Part print with two shaded views. Sizes in mm from the minimum x, y, z corner. A direction names the side the tool comes from. Coordinates: 2 decimals unless noted, no trailing zeros. Write each loop counter-clockwise with the first axis right and the second up, starting at its lowest first coordinate (ties: lowest second). Pieces come first, ordered by that corner, then holes. Notation, with made-up numbers: (11.5, 57.5) -> (67.5, 57.5) arc R23 ccw to (67.5, 69.5) -> close; hole circle Ø10 at (53.25, 25.25). An arc over 180 degrees is marked (long way). Write item = value, one per line. Start each with the question number.
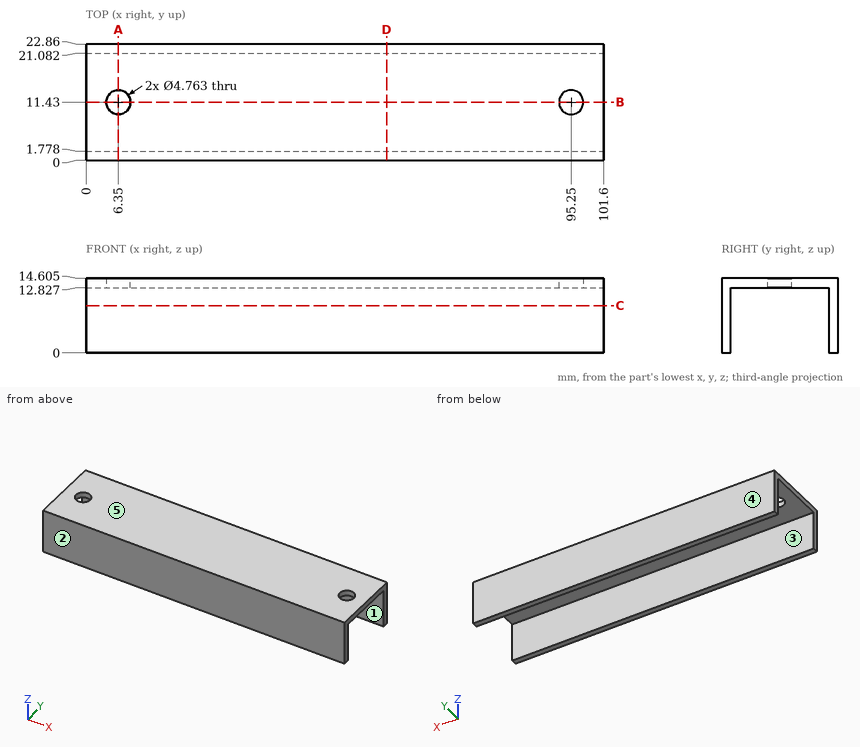
(1) 3-axis set-ups, long thin cutter, end or side, ignore diameter. For the marked faces 1 and 2: which of +Z, -Z, +X, -X, +Y, -Y reach the whole face in a straight line?
(2) Saw through at A-A (x = 6.35). Give the cut face in (y, z) (1 decimal).
(3) Saw through at B-B (y = 11.43). Give the cut face in (x, z) (1 decimal).
(4) Drop a flat-ended pin along its axis: pin 1 Ø5 at (x, y) = (65.5, 9.5) entering from -Z. Give the stop position or say it passes through.
(5) Saw through at D-D (x = 59). Give the cut face in (y, z) (1 decimal).
(6) Saw through at C-C (z = 9.25). Give the cut face in (x, y).
(7) Mould opens along Y. For the marked faces 3, 4 and 5 say: released by +Y, released by -Y, zero draft, split by the parting line, or undercut.
(8) Drill centre lines: line 1 along Y through (x, z) = (6.35, 14.2); line 2 along Y through (x, z) = (32.5, 7); line 3 along Z through (x, y) = (10, 9.75) (1 decimal). Where is each one in solid material? Low to high.
Returned:
q1.face_1 = -Z, +X, -X
q1.face_2 = +Z, -Z, +X, -X, -Y
q2.outline = (0, 0) -> (1.8, 0) -> (1.8, 12.8) -> (9, 12.8) -> (9, 14.6) -> (0, 14.6) -> close; (13.8, 12.8) -> (21.1, 12.8) -> (21.1, 0) -> (22.9, 0) -> (22.9, 14.6) -> (13.8, 14.6) -> close
q3.outline = (0, 12.8) -> (4, 12.8) -> (4, 14.6) -> (0, 14.6) -> close; (8.7, 12.8) -> (92.9, 12.8) -> (92.9, 14.6) -> (8.7, 14.6) -> close; (97.6, 12.8) -> (101.6, 12.8) -> (101.6, 14.6) -> (97.6, 14.6) -> close
q4.pin_1 = 12.83
q5.outline = (0, 0) -> (1.8, 0) -> (1.8, 12.8) -> (21.1, 12.8) -> (21.1, 0) -> (22.9, 0) -> (22.9, 14.6) -> (0, 14.6) -> close
q6.outline = (0, 0) -> (101.6, 0) -> (101.6, 1.78) -> (0, 1.78) -> close; (0, 21.08) -> (101.6, 21.08) -> (101.6, 22.86) -> (0, 22.86) -> close
q7.face_3 = undercut
q7.face_4 = released by +Y
q7.face_5 = zero draft
q8.line_1 = 0 to 9.05, 13.81 to 22.86
q8.line_2 = 0 to 1.78, 21.08 to 22.86
q8.line_3 = 12.8 to 14.6
